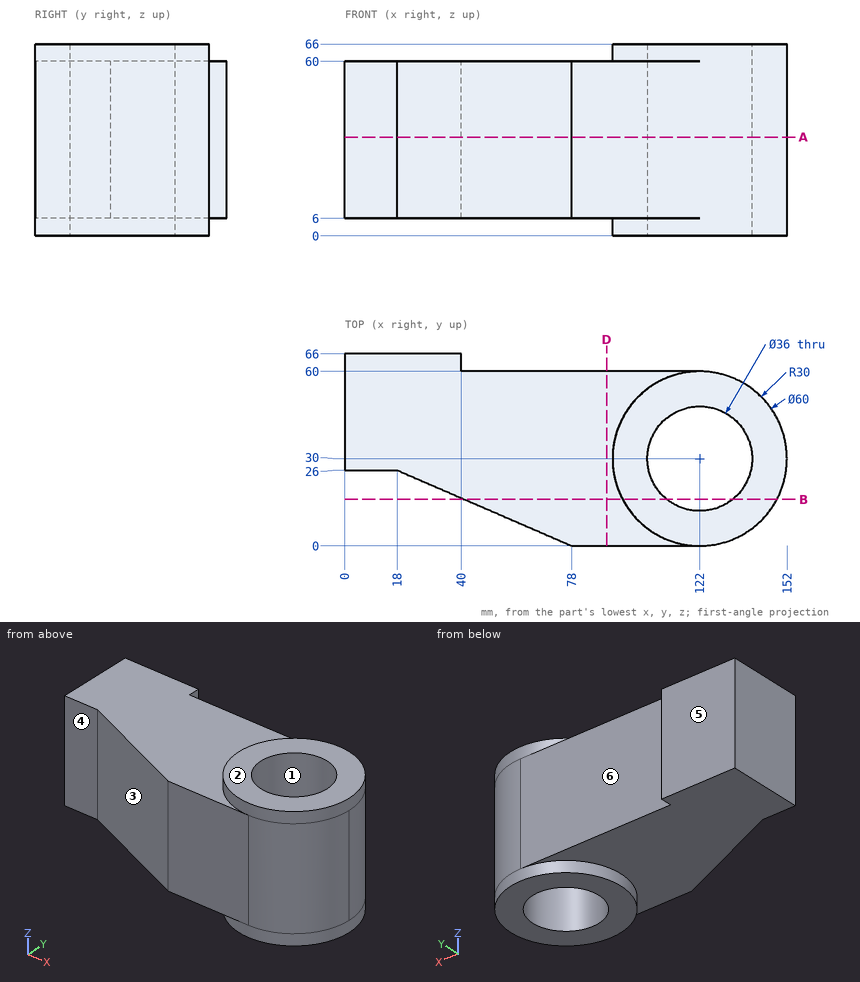
Here's the drawing with two shaded views (mm, measured from the low corner). I have some questions. A direction names the side the tool comes from. Give positions to 0.01 mm unless a question says otherwise; leave off trailing zeros. Loops run counter-clockwise (first coordinate to the right, second up) from the corner with the lowest first, then second, coordinate; pieces in that order, holes last. Notation, with made-up numbers: M 7.5,53 L 46.5,53 A29 cw 46.5,78 Z; hole C -40,-24.5 d9. An arc over 180 degrees is marked long. One line per item, written item: value.
1) I'm going to push flat-ended pins straight in: pin 1 (1.8 mm diameter, centred on y = 62, z = 20, fed in from +X); pin 2 (16 mm diameter, centred on x = 93, z = 23.5, fed in from +Y); pin 3 (20 mm diameter, centred on x = 45.5, y = 23, fed in from -Z). Where does each tip first touch, or does it pass through?
Geometry check:
pin 1: stops at x = 40
pin 2: stops at y = 60
pin 3: stops at z = 6
2) Imagine slicing it at A-A on z = 34. Write out the boundary of the cut face in (x, y), and give its area (3 significant figures).
Geometry check:
outline: M 0,26 L 18,26 L 78,0 L 122,0 A30 ccw 122,60 L 40,60 L 40,66 L 0,66 Z; hole C 122,30 d36
area: 6,710 mm²
3) Imagine slicing it at D-D on x = 90. Write out the boundary of the cut face in (y, z).
Geometry check:
outline: M 0,6 L 60,6 L 60,60 L 0,60 Z
4) Imagine slicing it at B-B on y = 16. Write out the boundary of the cut face in (x, z), and give its area (3 significant figures).
Geometry check:
outline: M 41.08,6 L 95.47,6 L 95.47,0 L 110.69,0 L 110.69,66 L 95.47,66 L 95.47,60 L 41.08,60 Z; M 133.31,0 L 148.53,0 L 148.53,66 L 133.31,66 Z
area: 4,950 mm²
5) Thinking about a two-plate mould opening in X: for the marked faces 1, 2 and 3, which applies, +X half, -X half, draft (parallel to the pull), parting line (faces both ways), or undercut?
Geometry check:
face 1: undercut
face 2: draft
face 3: -X half
6) On a 3-axis mill with a long thin cutter (end or side, diameter ignored), from which of +Z, -Z, +X, -X, +Y, -Y can I reach the whole of each face in a straight line? I mean the marked faces 4, 5 and 6. Say none if no direction works.
Geometry check:
face 4: +Z, -Z, -X, -Y
face 5: +Z, -Z, +X, -X, +Y
face 6: +Z, -Z, +X, +Y
7) Please list where these lines run through material, in increasing order: line 1 (X direction, y = 30.5, z = 52); line 2 (Y direction, x = 122, z = 51.5); line 3 (Z direction, x = 80, y = 56).
Geometry check:
line 1: x = 0 to 104.01, 139.99 to 152
line 2: y = 0 to 12, 48 to 60
line 3: z = 6 to 60
